from build123d import *

# Parameters (mm, degrees)
SKETCH1_W           = 13.462
SKETCH1_H           = 69.85
BOSS_EXTRUDE1_DEPTH = 4.9609375
SKETCH2_W           = 4.9609375
SKETCH2_H           = 7.62
BOSS_EXTRUDE2_DEPTH = 21.59
SKETCH3_OUTSIDE_W   = 52.714
SKETCH3_OUTSIDE_H   = 87.512
CUT_EXTRUDE1_DEPTH  = 5.9609375


with BuildPart() as part:
    # Sketch1 → Boss-Extrude1 (new body)
    with BuildSketch(Plane.XY):
        Rectangle(SKETCH1_W, SKETCH1_H)
    extrude(amount=BOSS_EXTRUDE1_DEPTH)

    # Sketch2 → Boss-Extrude2 (add)
    with BuildSketch(Plane(origin=(6.731, 0, 0), x_dir=(0, 0, -1), z_dir=(1, 0, 0))):
        with Locations((-2.48046875, 31.115)):
            Rectangle(SKETCH2_W, SKETCH2_H)
    extrude(amount=BOSS_EXTRUDE2_DEPTH)

    # Sketch3 outside → Cut-Extrude1 (cut, through all)
    with BuildSketch(Plane.XY.offset(4.9609375)):
        with Locations((10.795, 0)):
            Rectangle(SKETCH3_OUTSIDE_W, SKETCH3_OUTSIDE_H)
        Polygon((6.731, -34.925), (6.731, 27.305), (28.321, 27.305), (28.321, 34.925), (-6.731, 34.925), (-6.731, -34.925), align=None, mode=Mode.SUBTRACT)
        with BuildLine():
            Line((-1.825, -29.157786744), (-1.825, -25.451373384))
            ThreePointArc((-1.825, -25.451373384), (-1.79628168, -25.323286499), (-1.715625, -25.219722549))
            ThreePointArc((-1.715625, -25.219722549), (0, -24.604580064), (1.715625, -25.219722549))
            ThreePointArc((1.715625, -25.219722549), (1.79628168, -25.323286499), (1.825, -25.451373384))
            Line((1.825, -25.451373384), (1.825, -29.157786744))
            ThreePointArc((1.825, -29.157786744), (1.79628168, -29.285873629), (1.715625, -29.389437579))
            ThreePointArc((1.715625, -29.389437579), (0, -30.004580064), (-1.715625, -29.389437579))
            ThreePointArc((-1.715625, -29.389437579), (-1.79628168, -29.285873629), (-1.825, -29.157786744))
        make_face()
    extrude(amount=-CUT_EXTRUDE1_DEPTH, mode=Mode.SUBTRACT)


solid = part.part
Work out the finished part from the listing and answer in its coordinate system (mm). A direction names the side the tool comes from. Coordinates: 2 decimals unless noted, no trailing zeros. Write each loop counter-clockwise with the first axis right and the second up, starting at its lowest first coordinate (ties: lowest second). Pieces come first, ordered by that corner, then holes. Notation, with made-up numbers: M -2.75,34.25 L 54.25,34.25 A6 ccw 54.25,40.25 Z; hole C 87,58 d7. An arc over 180 degrees is marked long. Answer as CSV lines item,"result". Start each with the question number.
Item 1: Section A-A on x = 0.5 is taken. Write down the section's boundary in (y, z) (3 decimals), and give its area (3 significant figures).
Item 2: Flat-ended cylindrical pins translate along their axes: P1, Ø2.5, axis at x = 13.5, z = 3, coming from the -Y side (3 decimals); P2, Ø1.5, axis at y = -14.5, z = 4.5, coming from the +X side. Find the tip coordinate at first contact, or state that the pin passes through.
Item 3: Section B-B on z = 1.2 is taken. Write down the section's boundary in (x, y) (3 decimals), and give its area (3 significant figures).
Item 4: Consider L1, parallel to X at y = -26.5, z = 3.65 (3 decimals); L2, parallel to X at y = -9, z = 1.2; L3, parallel to Y at x = 15, z = 2.2 (3 decimals). Determine where each line is inside the solid, lowest interval first.
Item 5: Determine the mould class of faces 4 (the face through (-0.026, -24.605, 2.515)), 5 (the face through (11, 34.925, 3)), 6 (the face through (-6.731, 0, 2)), 7 (the face through (28.321, 31, 3)) for opening direction X: released by +X, released by -X, zero draft, split by the parting line, or undercut.
Item 6: Section D-D on x = 18 is taken. Write down the section's boundary in (y, z) (3 decimals).
Item 7: Section C-C on y = -6 is taken. Write down the section's boundary in (x, z), and give its area (3 significant figures).
Item 8: A tool of negligible diameter and unlimited length cuts with its end or side. For faces 1 (the face through (1.825, -27, 3)), 2 (the face through (6.731, -4, 2)), 3 (the face through (0, -34.925, 2)), from which of +Z, -Z, +X, -X, +Y, -Y can it reach the whole face along a straight path? Write none if from no direction.
Checks:
1,outline,"M -34.925,0 L -29.958,0 L -29.958,4.961 L -34.925,4.961 Z; M -24.651,0 L 34.925,0 L 34.925,4.961 L -24.651,4.961 Z"
1,area,"320 mm²"
2,P1,"stops at y = 27.305"
2,P2,"stops at x = 6.73"
3,outline,"M -6.731,-34.925 L 6.731,-34.925 L 6.731,27.305 L 28.321,27.305 L 28.321,34.925 L -6.731,34.925 Z; hole M -1.825,-29.158 A0.3 ccw -1.716,-29.389 A2.7 ccw 1.716,-29.389 A0.3 ccw 1.825,-29.158 L 1.825,-25.451 A0.3 ccw 1.716,-25.22 A2.7 ccw -1.716,-25.22 A0.3 ccw -1.825,-25.451 Z"
3,area,"1,090 mm²"
4,L1,"x = -6.731 to -1.825, 1.825 to 6.731"
4,L2,"x = -6.73 to 6.73"
4,L3,"y = 27.305 to 34.925"
5,face 4,"undercut"
5,face 5,"zero draft"
5,face 6,"released by -X"
5,face 7,"released by +X"
6,outline,"M 27.305,0 L 34.925,0 L 34.925,4.961 L 27.305,4.961 Z"
7,outline,"M -6.73,0 L 6.73,0 L 6.73,4.96 L -6.73,4.96 Z"
7,area,"66.8 mm²"
8,face 1,"+Z, -Z"
8,face 2,"+Z, -Z, +X, -Y"
8,face 3,"+Z, -Z, +X, -X, -Y"
